Check sheet for the modelled part. Datum: model origin and axes. Units: mm. Give positions to 0.01 mm unless a question says otherwise; leave off trailing zeros. Loops run counter-clockwise (first coordinate to the right, second up) from the corner with the lowest first, then second, coordinate; pieces in that order, holes last. Notation, with made-up numbers: (-33, 55) - (5, 55) arc R25 cw to (5, 75) - close; hole circle Ø6 at (-28.5, 31.5). An arc over 180 degrees is marked (long way). Answer in a Markdown table with one row per item. Add a question column.
(1) Sectioned sample at C-C on y = 1. Enter the section's corners in (x, z).
(2) Sectioned sample at D-D on x = -24. Enter the section's corners in (y, z), then the cut area to 3 significant figures.
(3) Go/stop test with flat-tipped pins: P1, Ø4, axis at x = 10, z = 1, coming from the -Y side; P2, Ø18, axis at x = -24.75, y = -14.29, coming from the +Z side; P3, Ø3, axis at x = -29, z = -2.5, coming from the +Y side. Record where each tip stops, or that it passes through.
(4) Sectioned sample at A-A on z = 1.5. Enter the section's corners in (x, y) (1 decimal), then the cut area to 3 significant figures.
(5) Draft check along Y on faces 1 (the face through (15.45, 8.65, -0.05)), 2 (the face through (-6, 10, -3.505)). Enter one of: released by +Y, released by -Y, zero draft, split by the parting line, or undercut.
(6) Thickness scan on L1, parallel to X at y = -15, z = -1; L2, parallel to X at y = -21, z = 3; L3, parallel to X at y = -8.5, z = 1.5. Record the ranges inside material, lowest first.
(7) Sectioned sample at B-B on x = 0. Enter the section's corners in (y, z) (3 decimals).
from build123d import *

# Parameters (mm, degrees)
F1_DEPTH = 3.5052


with BuildPart() as f1:
    # F0 (on Top) → F1 (new body, symmetric)
    with BuildSketch(Plane.XY):
        with BuildLine():
            ThreePointArc((10.9123688672, 26.4092944), (12.2452222147, 25.8183105162), (13.5461962881, 25.1601111111))
            ThreePointArc((13.5461962881, 25.1601111111), (13.8636442205, 26.8544567929), (13.97, 28.575))
            ThreePointArc((13.97, 28.575), (-1.7205432071, 42.4386442205), (-13.5461962881, 25.1601111111))
            ThreePointArc((-13.5461962881, 25.1601111111), (-12.2452222147, 25.8183105162), (-10.9123688672, 26.4092944))
            ThreePointArc((-10.9123688672, 26.4092944), (-1.0880691427, 39.6468643679), (11.1252, 28.575))
            ThreePointArc((11.1252, 28.575), (11.0718643679, 27.4869308573), (10.9123688672, 26.4092944))
        make_face()
        with BuildLine():
            ThreePointArc((13.4157103354, 24.6788973069), (13.4831003065, 24.9189220298), (13.5461962881, 25.1601111111))
            ThreePointArc((13.5461962881, 25.1601111111), (12.2452222147, 25.8183105162), (10.9123688672, 26.4092944))
            ThreePointArc((10.9123688672, 26.4092944), (0, 17.4498), (-10.9123688672, 26.4092944))
            ThreePointArc((-10.9123688672, 26.4092944), (-12.2452222147, 25.8183105162), (-13.5461962881, 25.1601111111))
            ThreePointArc((-13.5461962881, 25.1601111111), (-13.4831003065, 24.9189220298), (-13.4157103354, 24.6788973069))
            ThreePointArc((-13.4157103354, 24.6788973069), (0, 14.605), (13.4157103354, 24.6788973069))
        make_face()
        with BuildLine():
            ThreePointArc((28.0804071729, -0.7211026931), (15.3318346185, 8.8518388441), (13.4157103354, 24.6788973069))
            ThreePointArc((13.4157103354, 24.6788973069), (0, 14.605), (-13.4157103354, 24.6788973069))
            ThreePointArc((-13.4157103354, 24.6788973069), (-15.3318346185, 8.8518388441), (-28.0804071729, -0.7211026931))
            ThreePointArc((-28.0804071729, -0.7211026931), (-19.2663983542, -1.4373070879), (-12.6483010223, -7.3025))
            Line((-12.6483010223, -7.3025), (-9.6347058222, -5.5626))
            ThreePointArc((-9.6347058222, -5.5626), (-2.8794136406, 10.7461180026), (11.1252, 0))
            ThreePointArc((11.1252, 0), (10.7461180026, -2.8794136406), (9.6347058222, -5.5626))
            Line((9.6347058222, -5.5626), (12.6483010223, -7.3025))
            ThreePointArc((12.6483010223, -7.3025), (19.2663983542, -1.4373070879), (28.0804071729, -0.7211026931))
        make_face()
        with BuildLine():
            ThreePointArc((28.32730428, -3.7542585455), (28.4819238972, -2.3044817452), (28.5623935283, -0.8487054454))
            ThreePointArc((28.5623935283, -0.8487054454), (28.321969666, -0.7827536277), (28.0804071729, -0.7211026931))
            ThreePointArc((28.0804071729, -0.7211026931), (19.2663983542, -1.4373070879), (12.6483010223, -7.3025))
            Line((12.6483010223, -7.3025), (15.111970091, -8.7249))
            ThreePointArc((15.111970091, -8.7249), (20.8300724642, -3.8745132784), (28.32730428, -3.7542585455))
        make_face()
        with BuildLine():
            ThreePointArc((38.7166759131, -14.2875), (35.8926723936, -5.8656437641), (28.5623935283, -0.8487054454))
            ThreePointArc((28.5623935283, -0.8487054454), (28.4819238972, -2.3044817452), (28.32730428, -3.7542585455))
            ThreePointArc((28.32730428, -3.7542585455), (33.7911571516, -7.8092722974), (35.8718759131, -14.2875))
            ThreePointArc((35.8718759131, -14.2875), (29.3403125785, -24.4200503812), (17.4149354128, -22.6550358545))
            ThreePointArc((17.4149354128, -22.6550358545), (16.2367016825, -23.513828771), (15.0161972402, -24.3114056657))
            ThreePointArc((15.0161972402, -24.3114056657), (30.1884638978, -27.1540396875), (38.7166759131, -14.2875))
        make_face()
        with BuildLine():
            ThreePointArc((17.4149354128, -22.6550358545), (13.7704631585, -16.1021152775), (15.111970091, -8.7249))
            Line((15.111970091, -8.7249), (12.6483010223, -7.3025))
            ThreePointArc((12.6483010223, -7.3025), (10.8779436283, -15.9665368702), (14.6646968374, -23.9577946137))
            ThreePointArc((14.6646968374, -23.9577946137), (14.8388693595, -24.1361684021), (15.0161972402, -24.3114056657))
            ThreePointArc((15.0161972402, -24.3114056657), (16.2367016825, -23.513828771), (17.4149354128, -22.6550358545))
        make_face()
        with BuildLine():
            ThreePointArc((14.6646968374, -23.9577946137), (10.8779436283, -15.9665368702), (12.6483010223, -7.3025))
            Line((12.6483010223, -7.3025), (9.6347058222, -5.5626))
            ThreePointArc((9.6347058222, -5.5626), (0, -11.1252), (-9.6347058222, -5.5626))
            Line((-9.6347058222, -5.5626), (-12.6483010223, -7.3025))
            ThreePointArc((-12.6483010223, -7.3025), (-11.2526921199, -10.6717979399), (-10.7766759131, -14.2875))
            ThreePointArc((-10.7766759131, -14.2875), (-11.7850759408, -19.498817123), (-14.6646968374, -23.9577946137))
            ThreePointArc((-14.6646968374, -23.9577946137), (0, -17.7036776883), (14.6646968374, -23.9577946137))
        make_face()
        with BuildLine():
            ThreePointArc((-17.4149354128, -22.6550358545), (-16.2367016825, -23.513828771), (-15.0161972402, -24.3114056657))
            ThreePointArc((-15.0161972402, -24.3114056657), (-14.8388693595, -24.1361684021), (-14.6646968374, -23.9577946137))
            ThreePointArc((-14.6646968374, -23.9577946137), (-11.7850759408, -19.498817123), (-10.7766759131, -14.2875))
            ThreePointArc((-10.7766759131, -14.2875), (-11.2526921199, -10.6717979399), (-12.6483010223, -7.3025))
            Line((-12.6483010223, -7.3025), (-15.111970091, -8.7249))
            ThreePointArc((-15.111970091, -8.7249), (-14.0005579105, -11.4080863594), (-13.6214759131, -14.2875))
            ThreePointArc((-13.6214759131, -14.2875), (-14.614125532, -18.8811366653), (-17.4149354128, -22.6550358545))
        make_face()
        with BuildLine():
            ThreePointArc((-12.6483010223, -7.3025), (-19.2663983542, -1.4373070879), (-28.0804071729, -0.7211026931))
            ThreePointArc((-28.0804071729, -0.7211026931), (-28.321969666, -0.7827536277), (-28.5623935283, -0.8487054454))
            ThreePointArc((-28.5623935283, -0.8487054454), (-28.4819238972, -2.3044817452), (-28.32730428, -3.7542585455))
            ThreePointArc((-28.32730428, -3.7542585455), (-20.8300724642, -3.8745132784), (-15.111970091, -8.7249))
            Line((-15.111970091, -8.7249), (-12.6483010223, -7.3025))
        make_face()
        with BuildLine():
            ThreePointArc((-28.32730428, -3.7542585455), (-28.4819238972, -2.3044817452), (-28.5623935283, -0.8487054454))
            ThreePointArc((-28.5623935283, -0.8487054454), (-36.845050804, -21.2725), (-15.0161972402, -24.3114056657))
            ThreePointArc((-15.0161972402, -24.3114056657), (-16.2367016825, -23.513828771), (-17.4149354128, -22.6550358545))
            ThreePointArc((-17.4149354128, -22.6550358545), (-34.3813817353, -19.8501), (-28.32730428, -3.7542585455))
        make_face()
    extrude(amount=F1_DEPTH, both=True)


solid = f1.part
Reply:
| question | item | result |
|---|---|---|
| 1 | outline | (-23.52, -3.51) - (-11.08, -3.51) - (-11.08, 3.51) - (-23.52, 3.51) - close; (11.08, -3.51) - (23.52, -3.51) - (23.52, 3.51) - (11.08, 3.51) - close |
| 2 | outline | (-28.24, -3.51) - (-25.39, -3.51) - (-25.39, 3.51) - (-28.24, 3.51) - close; (-3.19, -3.51) - (0.76, -3.51) - (0.76, 3.51) - (-3.19, 3.51) - close |
| 2 | area | 47.6 mm^2 |
| 3 | P1 | y = -21.63 |
| 3 | P2 | through |
| 3 | P3 | y = -0.57 |
| 4 | outline | (-28.1, -0.7) arc R14 ccw (long way) to (-14.7, -24) arc R20.3 cw to (14.7, -24) arc R14 ccw (long way) to (28.1, -0.7) arc R20.3 cw to (13.4, 24.7) arc R14 ccw (long way) to (-13.4, 24.7) arc R20.3 cw to start; hole circle Ø22.3 at (-24.7, -14.3); hole circle Ø22.3 at (0, 0); hole circle Ø22.3 at (0, 28.6); hole circle Ø22.3 at (24.7, -14.3) |
| 4 | area | 1,350 mm^2 |
| 5 | face 1 | undercut |
| 5 | face 2 | zero draft |
| 6 | L1 | -38.7 to -35.85, -13.64 to 13.64, 35.85 to 38.7 |
| 6 | L2 | -37 to -33.62, -15.87 to -11.09, 11.09 to 15.87, 33.62 to 37 |
| 6 | L3 | -37.46 to -34.25, -15.25 to -7.18, 7.18 to 15.25, 34.25 to 37.46 |
| 7 | outline | (-17.704, -3.505) - (-11.125, -3.505) - (-11.125, 3.505) - (-17.704, 3.505) - close; (11.125, -3.505) - (17.45, -3.505) - (17.45, 3.505) - (11.125, 3.505) - close; (39.7, -3.505) - (42.545, -3.505) - (42.545, 3.505) - (39.7, 3.505) - close |
